from build123d import *

# Parameters (mm, degrees)
PAD_DEPTH    = 50
POCKET_DEPTH = 10


with BuildPart() as part:
    # Sketch → Pad (new body)
    with BuildSketch(Plane.XY):
        with BuildLine():
            Line((0, 0), (8, 0))
            ThreePointArc((8, 0), (24.970563, 7.029437), (32, 24))
            Line((32, 24), (32, 83))
            Line((32, 83), (0, 83))
            Line((0, 83), (0, 0))
        make_face()
    extrude(amount=PAD_DEPTH)

    # Sketch001 (on Face7 of Pad) → Pocket (cut)
    with BuildSketch(Plane.XY.offset(50)):
        with BuildLine():
            Line((3, 84), (3, 3))
            Line((3, 3), (8, 3))
            ThreePointArc((8, 3), (22.849242, 9.150758), (29, 24))
            Line((29, 24), (29, 84))
            Line((29, 84), (3, 84))
        make_face()
    extrude(amount=-POCKET_DEPTH, mode=Mode.SUBTRACT)


solid = part.part
Verification items for the finished model (mm, model axes). A direction names the side the tool comes from. Give positions to 0.01 mm unless a question says otherwise; leave off trailing zeros. Order: outer loops, then holes, each group sorted by start corner. A loop starts at its lowest first (then second) coordinate and runs counter-clockwise, first axis right, second up. Notation, with made-up numbers: M 28.5,10.5 L 42.5,10.5 A32 ccw 42.5,44.5 Z; hole C 52.25,-29 d11. An arc over 180 degrees is marked long. Use one line per item in the form item = value. Start each with the question number.
Q1. Section check B-B (z = 42). Enter the section's corners in (x, y), then the cut area to 3 significant figures.
Q2. Go/stop test with flat-tipped pins: pin 1 Ø6 at (x, y) = (12, 28) entering from +Z; pin 2 Ø8 at (x, z) = (13.5, 23.5) entering from -Y. Record where each tip stops, or that it passes through.
Q3. Scan lines: line 1 along Z through (x, y) = (14, 69); line 2 along Y through (x, z) = (4.5, 47); line 3 along Y through (x, z) = (15, 28). Record each from-to range of solid material in increasing order. Write a range as [from, to].
Q4. Section check D-D (z = 35). Enter the section's corners in (x, y).
Q5. Section check C-C (x = 4). Enter the section's corners in (y, z), then the cut area to 3 significant figures.
Q6. Access from +Z, -Z, +X, -X, +Y, -Y to the whole of each face (thin tool, end or side, straight path). Record for faces 4 (the flat face through (16, 83, 19)), 5 (the flat face through (16, 44, 40)).
Q7. Section check A-A (y = 66). Enter the section's corners in (x, z), then the cut area to 3 significant figures.
Q8. Mould release check, pull along X, two halves, no side actions. Record for faces 1 (the flat face through (0, 42, 25)), 2 (the flat face through (16, 42, 0)), 3 (the flat face through (3, 44, 45)): +X half, -X half, draft (parallel to the pull), parting line (faces both ways), or undercut.
Evaluation:
q1.outline = M 0,0 L 8,0 A24 ccw 32,24 L 32,83 L 29,83 L 29,24 A21 cw 8,3 L 3,3 L 3,83 L 0,83 Z
q1.area = 547 mm2
q2.pin_1 = 40
q2.pin_2 = 0.05
q3.line_1 = [0, 40]
q3.line_2 = [0, 3]
q3.line_3 = [1.04, 83]
q4.outline = M 0,0 L 8,0 A24 ccw 32,24 L 32,83 L 0,83 Z
q5.outline = M 0,0 L 83,0 L 83,40 L 3,40 L 3,50 L 0,50 Z
q5.area = 3,350 mm2
q6.face_4 = +Z, -Z, +X, -X, +Y
q6.face_5 = +Z, +Y
q7.outline = M 0,0 L 32,0 L 32,50 L 29,50 L 29,40 L 3,40 L 3,50 L 0,50 Z
q7.area = 1,340 mm2
q8.face_1 = -X half
q8.face_2 = draft
q8.face_3 = undercut
